For this review, use the dimensioned drawing (mm, ordinates from the lowest corner) and the shaded views. Coordinates: 2 decimals unless noted, no trailing zeros. Write each loop counter-clockwise with the first axis right and the second up, starting at its lowest first coordinate (ties: lowest second). Pieces come first, ordered by that corner, then holes. Notation, with made-up numbers: (-30, 1) - (21, 1) arc R8 cw to (21, 8) - close; hole circle Ø8 at (61.5, -6). An arc over 180 degrees is marked (long way). Use one line per item in the form item = value. Start each with the question number.
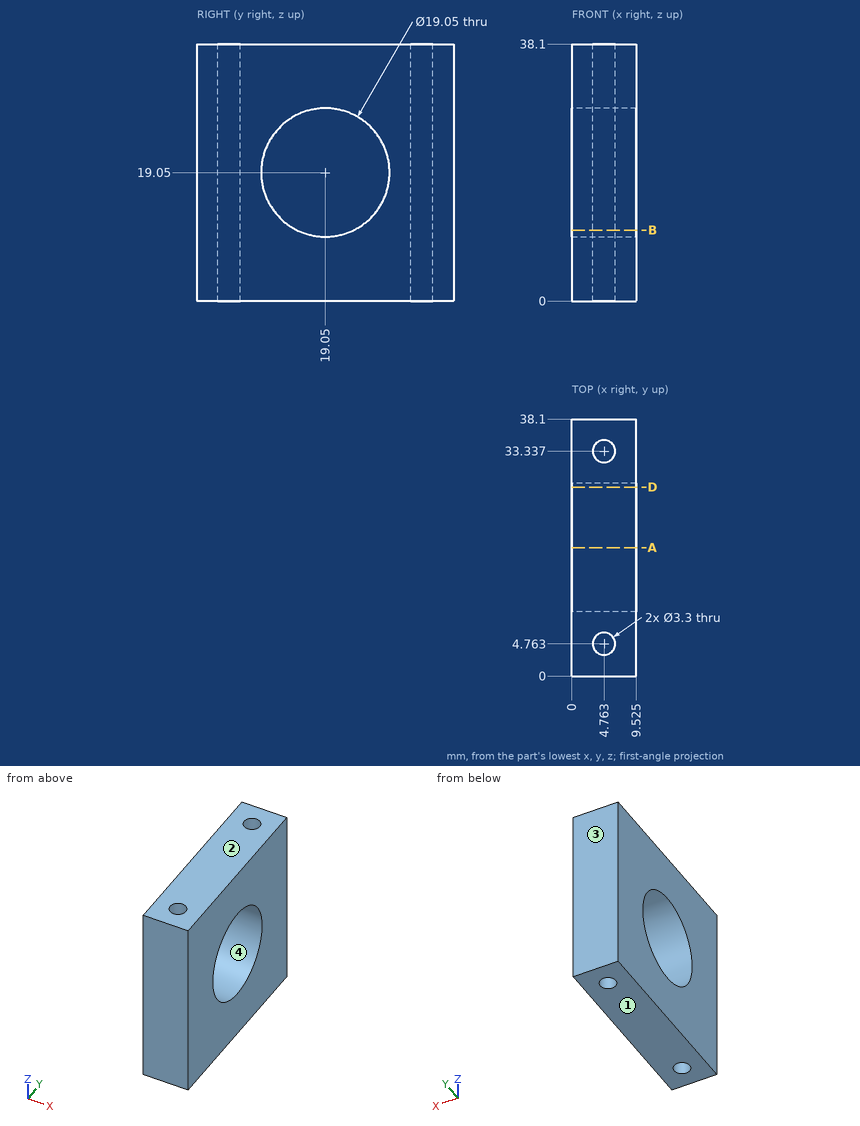
1. For L1, parallel to Y at x = 2.5, z = 19.5 (1 decimal); L2, parallel to Y at x = 8.75, z = 21.5 (1 decimal); L3, parallel to Y at x = 4.75, z = 22 (1 decimal), list the stretches that pass through material, from the lowest coordinate up.
2. Take a section at A-A (y = 19.05). State the section outline as (x, z) points (1 decimal).
3. Take a section at D-D (y = 28). State the section outline as (x, z) points (1 decimal), plus the area to 3 significant figures.
4. Take a section at B-B (z = 10.5). Count the separate pieces of the cut face and the enclosed holes in it, plus the area to 3 significant figures.
5. The part is to be moulded in two halves that separate along Z. For the marked faces 1, 2, 3 and 4, say which applies: released by +Z, released by -Z, zero draft, split by the parting line, or undercut.
6. For P1, Ø3, axis at x = 4.76, y = 33.34, coming from the -Z side, flat-tipped, find the tip position at first contact; note if it passes through.
Returned:
q1.L1 = 0 to 9.5, 28.6 to 38.1
q1.L2 = 0 to 9.8, 28.3 to 38.1
q1.L3 = 0 to 3.1, 6.4 to 10, 28.1 to 31.7, 35 to 38.1
q2.outline = (0, 0) - (9.5, 0) - (9.5, 9.5) - (0, 9.5) - close; (0, 28.6) - (9.5, 28.6) - (9.5, 38.1) - (0, 38.1) - close
q3.outline = (0, 0) - (9.5, 0) - (9.5, 15.8) - (0, 15.8) - close; (0, 22.3) - (9.5, 22.3) - (9.5, 38.1) - (0, 38.1) - close
q3.area = 301 mm²
q4.separate_pieces = 2
q4.enclosed_holes = 2
q4.area = 266 mm²
q5.face_1 = released by -Z
q5.face_2 = released by +Z
q5.face_3 = zero draft
q5.face_4 = undercut
q6.P1 = through
